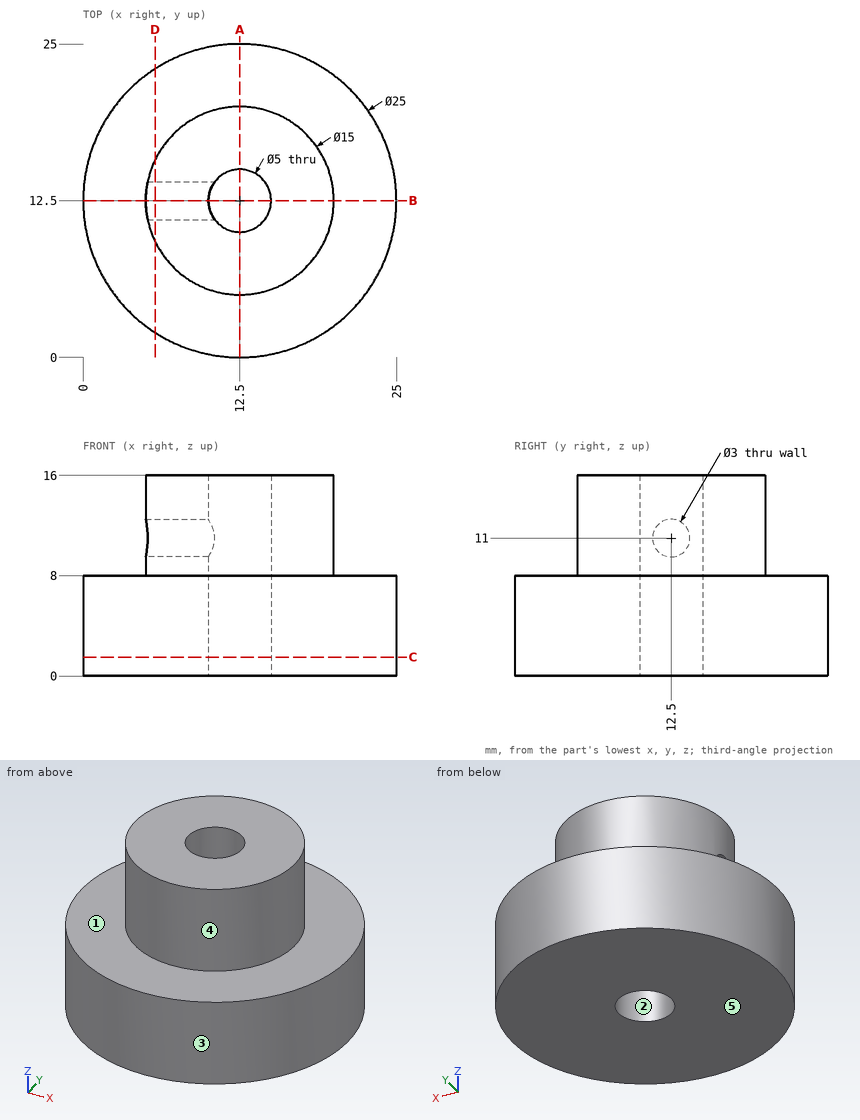
Verification items for this drawing (mm, ordinates from the low corner). A direction names the side the tool comes from. Give positions to 0.01 mm unless a question says otherwise; leave off trailing zeros. Write each loop counter-clockwise with the first axis right and the second up, starting at its lowest first coordinate (ties: lowest second). Pieces come first, ordered by that corner, then holes. Notation, with made-up numbers: (37, 25.25) -> (71, 25.25) arc R21 ccw to (71, 39.25) -> close; hole circle Ø7 at (23, 43). An arc over 180 degrees is marked (long way). Use CSV: the item, a comma, the result in double quotes. Start each with the question number.
Q1. Depth check by flat-ended pin: P1, Ø2.5, axis at y = 12.5, z = 11, coming from the -X side; P2, Ø2, axis at x = 14.5, z = 14, coming from the +Y side; P3, Ø6, axis at y = 5.5, z = 3, coming from the +X side. Enter the tip coordinate at first touch or a pass-through.
Q2. Cross-section at B-B on y = 12.5. Enter the section's corners in (x, z), and give its area (3 significant figures).
Q3. Cross-section at D-D on x = 5.75. Enter the section's corners in (y, z), and give its area (3 significant figures).
Q4. Tool access check on the marked faces 4 and 5. Record the directions out of +Z, -Z, +X, -X, +Y, -Y that give a thin tool (end or side, any length) a straight path to the whole face; none if there is none.
Q5. Release check for a two-part mould opening along X. For the marked faces 1, 2 and 3 record: +X half, -X half, draft (parallel to the pull), parting line (faces both ways), or undercut.
Q6. Scan lines: line 1 along Y through (x, z) = (12.5, 7.25); line 2 along Z through (x, y) = (7, 2.5); line 3 along Y through (x, z) = (11, 2). Record each from-to range of solid material in increasing order.
Q7. Cross-section at A-A on x = 12.5. Enter the section's corners in (y, z), and give its area (3 significant figures).
Q8. Cross-section at C-C on z = 1.5. Enter the section's corners in (x, y).
Working result:
1,P1,"stops at x = 14.67"
1,P2,"stops at y = 19.93"
1,P3,"stops at x = 24.34"
2,outline,"(0, 0) -> (10, 0) -> (10, 9.5) -> (5, 9.5) -> (5, 8) -> (0, 8) -> close; (5, 12.5) -> (10, 12.5) -> (10, 16) -> (5, 16) -> close; (15, 0) -> (25, 0) -> (25, 8) -> (20, 8) -> (20, 16) -> (15, 16) -> close"
2,area,"225 mm^2"
3,outline,"(1.98, 0) -> (23.02, 0) -> (23.02, 8) -> (15.77, 8) -> (15.77, 16) -> (9.23, 16) -> (9.23, 8) -> (1.98, 8) -> close; hole circle Ø3 at (12.5, 11)"
3,area,"214 mm^2"
4,face 4,"+Z"
4,face 5,"-Z, +X, -X, +Y, -Y"
5,face 1,"draft"
5,face 2,"undercut"
5,face 3,"parting line"
6,line 1,"y = 0 to 10, 15 to 25"
6,line 2,"z = 0 to 8"
6,line 3,"y = 0.09 to 10.5, 14.5 to 24.91"
7,outline,"(0, 0) -> (10, 0) -> (10, 16) -> (5, 16) -> (5, 8) -> (0, 8) -> close; (15, 0) -> (25, 0) -> (25, 8) -> (20, 8) -> (20, 16) -> (15, 16) -> close"
7,area,"240 mm^2"
8,outline,"circle Ø25 at (12.5, 12.5); hole circle Ø5 at (12.5, 12.5)"
